Source: CAD feature listing. Evaluate the final solid. Frame: model axes, mm. A direction names the side the tool comes from. Give positions to 0.01 mm unless a question says otherwise; leave off trailing zeros. Loops run counter-clockwise (first coordinate to the right, second up) from the corner with the lowest first, then second, coordinate; pieces in that order, holes last.
from build123d import *

# Parameters (mm, degrees)
BOSS_EXTRUDE1_DEPTH = 10
CUT_EXTRUDE1_DEPTH  = 6
SKETCH3_R           = 2.5
SKETCH3_R_2         = 1.6
CUT_EXTRUDE5_DEPTH  = 118.268793803
CUT_EXTRUDE6_DEPTH  = 3
FILLET1_R           = 10
SKETCH7_W           = 12
SKETCH7_H           = 3
CUT_EXTRUDE7_DEPTH  = 20


with BuildPart() as part:
    # Sketch1 → Boss-Extrude1 (new body)
    with BuildSketch(Plane(origin=(0, 0, 0), x_dir=(1, 0, 0), z_dir=(0, 1, 0))):
        with BuildLine():
            Line((-64.6, 70.6), (-13.781138102, 92.296857547))
            ThreePointArc((-13.781138102, 92.296857547), (-11.858510235, 92.897157125), (-9.854586018, 93.1))
            Line((-9.854586018, 93.1), (9.854586018, 93.1))
            ThreePointArc((9.854586018, 93.1), (11.858510235, 92.897157125), (13.781138102, 92.296857547))
            Line((13.781138102, 92.296857547), (64.6, 70.6))
            ThreePointArc((64.6, 70.6), (68.842640687, 68.842640687), (70.6, 64.6))
            Line((70.6, 64.6), (70.6, -64.6))
            ThreePointArc((70.6, -64.6), (68.842640687, -68.842640687), (64.6, -70.6))
            Line((64.6, -70.6), (-64.6, -70.6))
            ThreePointArc((-64.6, -70.6), (-68.842640687, -68.842640687), (-70.6, -64.6))
            Line((-70.6, -64.6), (-70.6, 64.6))
            ThreePointArc((-70.6, 64.6), (-68.842640687, 68.842640687), (-64.6, 70.6))
        make_face()
        with BuildLine():
            Line((-41, -54), (41, -54))
            ThreePointArc((41, -54), (50.192388155, -50.192388155), (54, -41))
            Line((54, -41), (54, 41))
            ThreePointArc((54, 41), (50.192388155, 50.192388155), (41, 54))
            Line((41, 54), (-41, 54))
            ThreePointArc((-41, 54), (-50.192388155, 50.192388155), (-54, 41))
            Line((-54, 41), (-54, -41))
            ThreePointArc((-54, -41), (-50.192388155, -50.192388155), (-41, -54))
        make_face(mode=Mode.SUBTRACT)
    extrude(amount=BOSS_EXTRUDE1_DEPTH)

    # Sketch2 → Cut-Extrude1 (cut)
    with BuildSketch(Plane(origin=(0, 10, 0), x_dir=(1, 0, 0), z_dir=(0, 1, 0))):
        with BuildLine():
            Line((-64.6, 68.6), (-11.9, 91.1))
            Line((-11.9, 91.1), (11.9, 91.1))
            Line((11.9, 91.1), (64.6, 68.6))
            ThreePointArc((64.6, 68.6), (67.428427125, 67.428427125), (68.6, 64.6))
            Line((68.6, 64.6), (68.6, -64.6))
            ThreePointArc((68.6, -64.6), (67.428427125, -67.428427125), (64.6, -68.6))
            Line((64.6, -68.6), (-64.6, -68.6))
            ThreePointArc((-64.6, -68.6), (-67.428427125, -67.428427125), (-68.6, -64.6))
            Line((-68.6, -64.6), (-68.6, 64.6))
            ThreePointArc((-68.6, 64.6), (-67.428427125, 67.428427125), (-64.6, 68.6))
        make_face()
        with BuildLine():
            Line((-41, -56), (41, -56))
            ThreePointArc((41, -56), (51.606601718, -51.606601718), (56, -41))
            Line((56, -41), (56, 41))
            ThreePointArc((56, 41), (51.606601718, 51.606601718), (41, 56))
            Line((41, 56), (-41, 56))
            ThreePointArc((-41, 56), (-51.606601718, 51.606601718), (-56, 41))
            Line((-56, 41), (-56, -41))
            ThreePointArc((-56, -41), (-51.606601718, -51.606601718), (-41, -56))
        make_face(mode=Mode.SUBTRACT)
    extrude(amount=-CUT_EXTRUDE1_DEPTH, mode=Mode.SUBTRACT)

    # Sketch3 → Cut-Extrude5 (cut, through all)
    with BuildSketch(Plane(origin=(0, 0, 0), x_dir=(1, 0, 0), z_dir=(0, 1, 0))):
        with Locations(Location((-64.6, 64.6, 0), (0, 0, 270))):
            Circle(SKETCH3_R)
        with Locations(Location((-48.6, 64.6, 0), (0, 0, 270))):
            Circle(SKETCH3_R)
        with Locations(Location((-55.87, 64.6, 0), (0, 0, 270))):
            Circle(SKETCH3_R_2)
        with Locations(Location((55.87, 64.6, 0), (0, 0, 90))):
            Circle(SKETCH3_R_2)
        with Locations(Location((48.6, 64.6, 0), (0, 0, 90))):
            Circle(SKETCH3_R)
        with Locations(Location((64.6, 64.6, 0), (0, 0, 90))):
            Circle(SKETCH3_R)
        with Locations(Location((64.6, -64.6, 0), (0, 0, 270))):
            Circle(SKETCH3_R)
        with Locations(Location((48.6, -64.6, 0), (0, 0, 270))):
            Circle(SKETCH3_R)
        with Locations(Location((55.87, -64.6, 0), (0, 0, 270))):
            Circle(SKETCH3_R_2)
        with Locations(Location((-55.87, -64.6, 0), (0, 0, 90))):
            Circle(SKETCH3_R_2)
        with Locations(Location((-48.6, -64.6, 0), (0, 0, 90))):
            Circle(SKETCH3_R)
        with Locations(Location((-64.6, -64.6, 0), (0, 0, 90))):
            Circle(SKETCH3_R)
    extrude(amount=CUT_EXTRUDE5_DEPTH, mode=Mode.SUBTRACT)

    # Sketch6 → Cut-Extrude6 (cut)
    with BuildSketch(Plane.XZ):
        Polygon((-52.405898385, 64.6), (-54.137949192, 67.6), (-57.602050808, 67.6), (-59.334101615, 64.6), (-57.602050808, 61.6), (-54.137949192, 61.6), align=None)
        Polygon((-54.137949192, -61.6), (-52.405898385, -64.6), (-54.137949192, -67.6), (-57.602050808, -67.6), (-59.334101615, -64.6), (-57.602050808, -61.6), align=None)
        Polygon((52.405898385, -64.6), (54.137949192, -67.6), (57.602050808, -67.6), (59.334101615, -64.6), (57.602050808, -61.6), (54.137949192, -61.6), align=None)
        Polygon((54.137949192, 61.6), (52.405898385, 64.6), (54.137949192, 67.6), (57.602050808, 67.6), (59.334101615, 64.6), (57.602050808, 61.6), align=None)
    extrude(amount=-CUT_EXTRUDE6_DEPTH, mode=Mode.SUBTRACT)

    # Fillet1
    fillet1_edges = [part.edges().sort_by_distance(p)[0] for p in [
        (-64.6, 5, -70.6),
        (64.6, 5, -70.6),
    ]]
    fillet(fillet1_edges, radius=FILLET1_R)

    # Sketch7 → Cut-Extrude7 (cut)
    with BuildSketch(Plane(origin=(0, 0, -93.1), x_dir=(-1, 0, 0), z_dir=(0, 0, -1))):
        with Locations((0, 2.73)):
            Rectangle(SKETCH7_W, SKETCH7_H)
    extrude(amount=-CUT_EXTRUDE7_DEPTH, mode=Mode.SUBTRACT)


solid = part.part
1) Ray query, probe 1 along Z at (x, y) = (-4.5, 6.5); probe 2 along X at (y, z) = (9, 29); probe 3 along X at (y, z) = (5.25, 46). Return the intervals inside material, ascending.
Checks:
probe 1: z = -93.1 to -91.1, -56 to -54, 54 to 56, 68.6 to 70.6
probe 2: x = -70.6 to -68.6, -56 to -54, 54 to 56, 68.6 to 70.6
probe 3: x = -70.6 to -68.6, -55.14 to -53, 53 to 55.14, 68.6 to 70.6
2) Pull-direction query (Z, two-part tool) for faces 1 (the cylindrical face through (-69.2, 4.93, -68.45)), 2 (the cylindrical face through (67.459, 7.042, 67.397)), 3 (the cylindrical face through (68.889, 4.93, 68.796)); classes: released by +Z, released by -Z, zero draft, split by the parting line, or undercut.
Checks:
face 1: released by -Z
face 2: undercut
face 3: released by +Z
3) Cut plane D-D (z = 59.5). Return loops of the section in (x, y).
Checks:
outline: (-70.6, 0) - (70.6, 0) - (70.6, 10) - (68.6, 10) - (68.6, 4) - (-68.6, 4) - (-68.6, 10) - (-70.6, 10) - close
4) Contact query for flat-ended pins moving along their axis: P1, Ø2.5, axis at x = 55.87, z = 64.6, coming from the +Y side; P2, Ø6.5, axis at x = 48.6, z = 64.6, coming from the -Y side; P3, Ø5, axis at x = 18, y = 4, coming from the -Z side; P4, Ø2.5, axis at y = 2.5, z = -80.5, coming from the -X side. Output: stop coordinate, or through.
Checks:
P1: passes through
P2: stops at y = 0
P3: stops at z = -91.56
P4: stops at x = -44.34
5) Cut plane A-A (z = 33.5). Return loops of the section in (x, y).
Checks:
outline: (-70.6, 0) - (-54, 0) - (-54, 10) - (-56, 10) - (-56, 4) - (-68.6, 4) - (-68.6, 10) - (-70.6, 10) - close; (54, 0) - (70.6, 0) - (70.6, 10) - (68.6, 10) - (68.6, 4) - (56, 4) - (56, 10) - (54, 10) - close
6) Cut plane B-B (y = 8). State how many separate pieces and enclosed holes the cut face has, and give its area (3 significant figures).
Checks:
separate pieces: 2
enclosed holes: 2
area: 1,930 mm2
7) Cut plane C-C (x = 48.6). Return loops of the section in (y, z), and give its area (3 significant figures).
Checks:
outline: (0, -77.43) - (10, -77.43) - (10, -75.43) - (4, -75.43) - (4, -67.1) - (0, -67.1) - close; (0, -62.1) - (4, -62.1) - (4, -53.93) - (10, -53.93) - (10, -51.55) - (0, -51.55) - close; (0, 51.55) - (10, 51.55) - (10, 53.93) - (4, 53.93) - (4, 62.1) - (0, 62.1) - close; (0, 67.1) - (4, 67.1) - (4, 68.6) - (10, 68.6) - (10, 70.6) - (0, 70.6) - close
area: 192 mm2
8) Reachability of faces 4 (the flat face through (1, 7, -56)), 5 (the flat face through (-54, 5, -1)), 6 (the flat face through (38.136, 4.93, -81.899)), 7 (the flat face through (1, 0, -67)), 8 (the flat face through (-54, 3, 65)) from +Z, -Z, +X, -X, +Y, -Y: full face, straight path, thin tool, end or side. Return the list, or none.
Checks:
face 4: +Y
face 5: +Y, -Y
face 6: -Z, +X, +Y, -Y
face 7: +Z, -Z, +X, -X, -Y
face 8: -Y
